Build history of the part. All positions in model axes, mm. Give positions to 0.01 mm unless a question says otherwise; leave off trailing zeros. Write each question's results on one line, items separated by ' | '. Start each with the question number.
1) Cut at A-A on x = 0. State how many separate pieces and enclosed holes the cut face has, plus the area to 3 significant figures.
2) Drill centre lines: line 1 along X through (y, z) = (0, 1.15); line 2 along X through (y, z) = (0, 5); line 3 along X through (y, z) = (14, 7). Where is each one in solid material? Low to high. Write a range as from..to.
3) Drop flat-ended pins along their axis: pin 1 Ø2 at (x, y) = (-13.5, 14) entering from -Z; pin 2 Ø6 at (x, z) = (13, 5.5) entering from +Y; pin 3 Ø1 at (y, z) = (-9.5, 3) entering from -X; pin 4 Ø2 at (x, z) = (-13, 8) entering from +Y. Give the stop position or say it passes through.
from build123d import *

# Parameters (mm, degrees)
SKETCH1_W                       = 10.668
SKETCH1_H                       = 12.7
SKETCH2_W                       = 0.762
SKETCH2_H                       = 0.762
LPATTERN1_COUNT                 = 10
LPATTERN1_PITCH                 = 1.0414
M4X0_7_TAPPED_HOLE1_D           = 4
M4X0_7_TAPPED_HOLE1_DEPTH       = 10.668
M4X0_7_TAPPED_HOLE1_CSINK_D     = 4.05
M4X0_7_TAPPED_HOLE1_CSINK_ANGLE = 90
CIRPATTERN1_COUNT               = 4


with BuildPart() as part:
    # Sketch1 → Revolve1 (revolve)
    with BuildSketch(Plane(origin=(0, 0, 0), x_dir=(0, 0, -1), z_dir=(1, 0, 0))):
        with Locations((-5.334, 14.9008)):
            Rectangle(SKETCH1_W, SKETCH1_H)
    revolve(axis=Axis((0, 0, 0), (0, 0, 1)))

    # Sketch2 → Cut-Revolve1 (revolve, cut)
    with BuildSketch(Plane(origin=(0, 0, 0), x_dir=(0, 0, -1), z_dir=(1, 0, 0))):
        with Locations((-0.635, 8.9318)):
            Rectangle(SKETCH2_W, SKETCH2_H)
    cut_revolve1 = revolve(axis=Axis((0, 0, 10.668), (0, 0, -1)), mode=Mode.SUBTRACT)

    # LPattern1: Cut-Revolve1 ×10
    with Locations(*[(0, 0, i * LPATTERN1_PITCH) for i in range(1, LPATTERN1_COUNT)]):
        add(cut_revolve1, mode=Mode.SUBTRACT)

    # M4x0.7 Tapped Hole1
    with Locations(Plane(origin=(0, 0, 0), x_dir=(-1, 0, 0), z_dir=(0, 0, -1))):
        with Locations((0, 14.478)):
            m4x0_7_tapped_hole1 = CounterSinkHole(M4X0_7_TAPPED_HOLE1_D / 2, M4X0_7_TAPPED_HOLE1_CSINK_D / 2, depth=M4X0_7_TAPPED_HOLE1_DEPTH, counter_sink_angle=M4X0_7_TAPPED_HOLE1_CSINK_ANGLE)

    # CirPattern1: M4x0.7 Tapped Hole1 ×4 about axis
    cirpattern1_axis = Axis((0, 0, 0), (0, 0, 1))
    for i in range(1, CIRPATTERN1_COUNT):
        add(m4x0_7_tapped_hole1.rotate(cirpattern1_axis, i * 360 / CIRPATTERN1_COUNT), mode=Mode.SUBTRACT)


solid = part.part
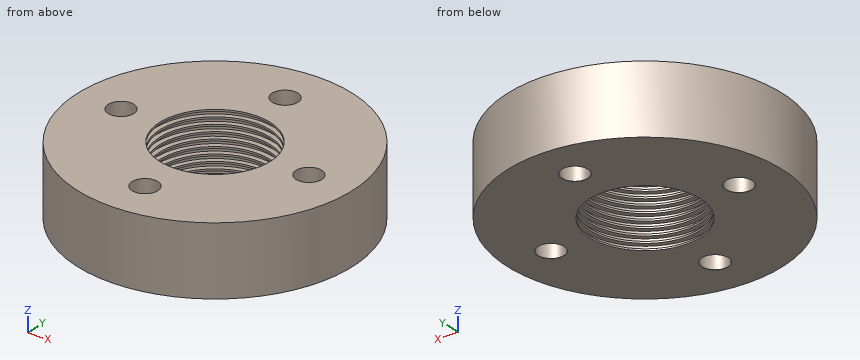
Results:
1) separate pieces: 4 | enclosed holes: 0 | area: 174 mm^2
2) line 1: -21.25..-16.48, -12.48..-8.55, 8.55..12.48, 16.48..21.25 | line 2: -21.25..-16.48, -12.48..-9.31, 9.31..12.48, 16.48..21.25 | line 3: -15.99..-1.94, 1.94..15.99
3) pin 1: z = 0 | pin 2: y = 18.75 | pin 3: x = -19.25 | pin 4: y = 17.54
